Read the model definition and answer for the solid it produces. Units are mm, in the model's axes. A direction names the side the tool comes from. Give positions to 0.01 mm unless a question says otherwise; leave off trailing zeros. Order: outer loops, then holes, each group sorted by start corner. A loop starts at its lowest first (then second) coordinate and runs counter-clockwise, first axis right, second up.
Item 1: A cutting plane is placed at B-B (x = 3.5). Write down the section's boundary in (y, z), plus the area to 3 significant figures.
Item 2: A cutting plane is placed at C-C (z = -0.1). State how many separate pieces and enclosed holes the cut face has, plus the area to 3 significant figures.
Item 3: Find the intervals of material crossed by line 1 along Y through (x, z) = (9.5, -0.6); line 2 along X through (y, z) = (-3, -0.95); line 3 along X through (y, z) = (21, -0.65), in increasing order.
Item 4: Given pin 1 Ø0.9 at (x, z) = (-27, 0) entering from +Y; pin 2 Ø1.5 at (x, z) = (-20.5, 0.5) entering from +Y; pin 3 Ø1.5 at (y, z) = (-36.5, 0.5) entering from +X, each flat-ended and moving along its own axis, determine where each tip first touches the part or whether it passes through.
Item 5: A cutting plane is placed at D-D (y = -22.5). Write down the section's boundary in (x, z).
Item 6: The mould has two halves that part along Y. Classify faces 6 (the face through (0, -43, 0)), 7 (the face through (-1, -37, 0)), 8 (the face through (25.5, -28, 0)): +Y half, -Y half, draft (parallel to the pull), parting line (faces both ways), or undercut.
Item 7: Which of the six approach directions +Z, -Z, +X, -X, +Y, -Y give full straight-line access (tool end or side, diameter ignored) to faces 1 (the face through (-25.5, 28, 0)), 2 (the face through (-28.5, 0, 0)), 3 (the face through (-4, -38, 0)), 4 (the face through (27, 15, 0)), 5 (the face through (-20, -40, 0))?
Item 8: A cutting plane is placed at A-A (x = -11). Write down the section's boundary in (y, z), plus the area to 3 significant figures.
from build123d import *

# Parameters (mm, degrees)
SKETCH1_W           = 30
SKETCH1_H           = 3
SKETCH1_W_2         = 5
BOSS_EXTRUDE1_DEPTH = 1.5


with BuildPart() as part:
    # Sketch1 → Boss-Extrude1 (new body, symmetric)
    with BuildSketch(Plane.XY):
        Polygon((-25.5, -15), (-25.5, -40), (-15, -40), (-15, -43), (15, -43), (15, -40), (25.5, -40), (25.5, -15), (28.5, -15), (28.5, 15), (25.5, 15), (25.5, 40), (15, 40), (15, 43), (-15, 43), (-15, 40), (-25.5, 40), (-25.5, 15), (-28.5, 15), (-28.5, -15), align=None)
        with Locations((0, -3.5)):
            Rectangle(SKETCH1_W, SKETCH1_H, mode=Mode.SUBTRACT)
        with Locations((3.5, -36.5)):
            Rectangle(SKETCH1_W_2, SKETCH1_H, mode=Mode.SUBTRACT)
        with Locations((-3.5, -36.5)):
            Rectangle(SKETCH1_W_2, SKETCH1_H, mode=Mode.SUBTRACT)
    extrude(amount=BOSS_EXTRUDE1_DEPTH, both=True)


solid = part.part
Response values:
1. outline: (-43, -1.5) - (-38, -1.5) - (-38, 1.5) - (-43, 1.5) - close; (-35, -1.5) - (-5, -1.5) - (-5, 1.5) - (-35, 1.5) - close; (-2, -1.5) - (43, -1.5) - (43, 1.5) - (-2, 1.5) - close
1. area: 240 mm2
2. separate pieces: 1
2. enclosed holes: 3
2. area: 4,320 mm2
3. line 1: y = -43 to -5, -2 to 43
3. line 2: x = -28.5 to -15, 15 to 28.5
3. line 3: x = -25.5 to 25.5
4. pin 1: stops at y = 15
4. pin 2: stops at y = 40
4. pin 3: stops at x = 25.5
5. outline: (-25.5, -1.5) - (25.5, -1.5) - (25.5, 1.5) - (-25.5, 1.5) - close
6. face 6: -Y half
6. face 7: undercut
6. face 8: draft
7. face 1: +Z, -Z, -X, +Y
7. face 2: +Z, -Z, -X, +Y, -Y
7. face 3: +Z, -Z
7. face 4: +Z, -Z, +X, +Y
7. face 5: +Z, -Z, -X, -Y
8. outline: (-43, -1.5) - (-5, -1.5) - (-5, 1.5) - (-43, 1.5) - close; (-2, -1.5) - (43, -1.5) - (43, 1.5) - (-2, 1.5) - close
8. area: 249 mm2
